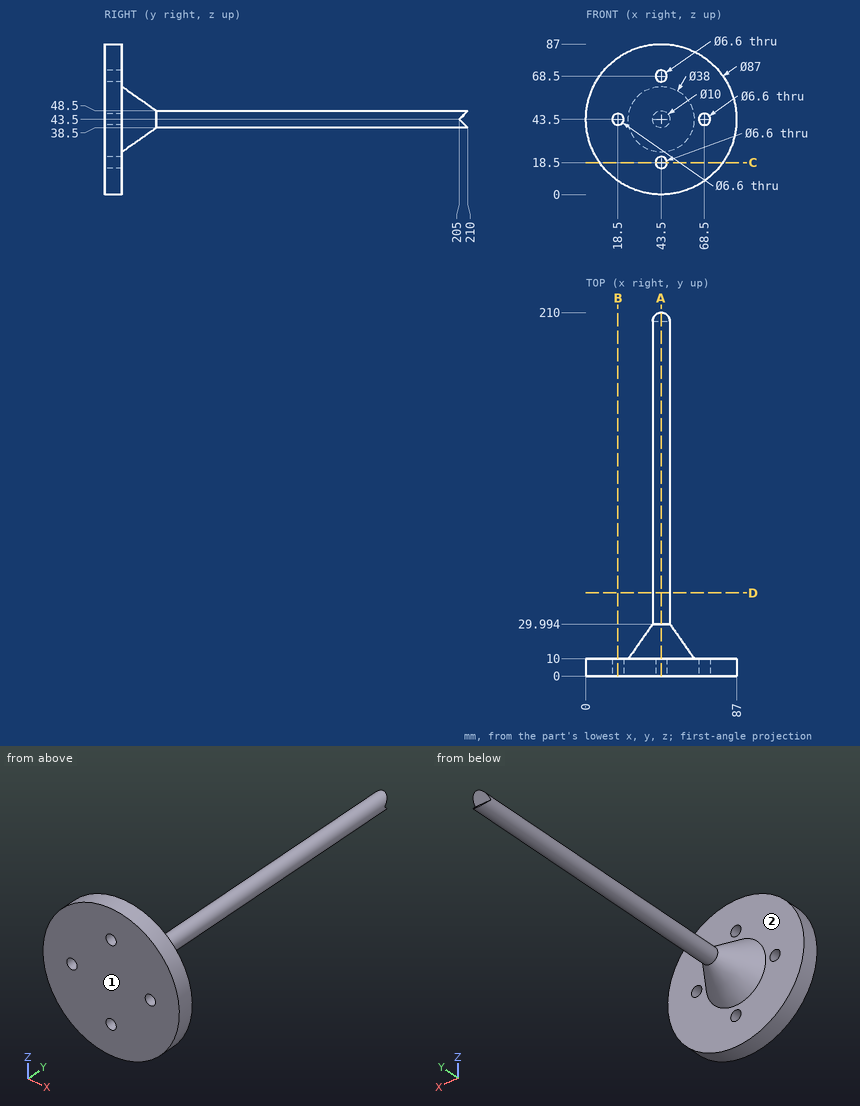
Answer from the drawing. Dimensions are ordinates in mm from the lowest x, y and z of the part. A direction names the side the tool comes from. Coordinates: 2 decimals unless noted, no trailing zeros. Order: outer loops, then holes, each group sorted by start corner. A loop starts at its lowest first (then second) coordinate and runs counter-clockwise, first axis right, second up. Notation, with made-up numbers: M 4,-23.75 L 51,-23.75 A28 cw 51,10.25 Z; hole C 61,-36.5 d1. An arc over 180 degrees is marked long. Put each result on its own line as item: value. Start each with the question number.
Item 1: For the marked faces 1 and 2, determine the directions among +Z, -Z, +X, -X, +Y, -Y from which every point of the face is accessible in a straight line to the end or side of a thin tool.
Item 2: Given pin 1 Ø1 at (x, z) = (73.5, 58) entering from +Y; pin 2 Ø10.5 at (x, z) = (68.5, 43.5) entering from -Y; pin 3 Ø5 at (y, z) = (48, 37.5) entering from -X; pin 4 Ø4 at (x, y) = (42.5, 57.5) entering from +Z, each flat-ended and moving along its own axis, determine where each tip first touches the part or whether it passes through.
Item 3: Section C-C, the plane z = 18.5 is taken. Determine the outline of the cut face in (x, y), plus the area to 3 significant figures.
Item 4: Section D-D, the plane y = 48 is taken. Determine the outline of the cut face in (x, z), plus the area to 3 significant figures.
Item 5: Section B-B, the plane x = 18.5 is taken. Determine the outline of the cut face in (y, z), plus the area to 3 significant figures.
Item 6: Consider probe 1 along Z at (x, y) = (43, 5); probe 2 along Y at (x, z) = (22, 28.5). Determine where each line is inside the solid, lowest interval first. Write a range as [from, to].
Item 7: Section A-A, the plane x = 43.5 is taken. Determine the outline of the cut face in (y, z).
Computed:
1. face 1: +Z, -Z, +X, -X, -Y
1. face 2: +Y
2. pin 1: stops at y = 10
2. pin 2: stops at y = 0
2. pin 3: stops at x = 39.93
2. pin 4: stops at z = 48.5
3. outline: M 7.9,0 L 40.2,0 L 40.2,10 L 7.9,10 Z; M 46.8,0 L 79.1,0 L 79.1,10 L 46.8,10 Z
3. area: 646 mm2
4. outline: C 43.5,43.5 d10
4. area: 78.5 mm2
5. outline: M 0,7.9 L 10,7.9 L 10,40.2 L 0,40.2 Z; M 0,46.8 L 10,46.8 L 10,79.1 L 0,79.1 Z
5. area: 646 mm2
6. probe 1: z = [0, 15.24], [21.76, 65.24], [71.76, 87]
6. probe 2: y = [0, 10]
7. outline: M 0,0 L 10,0 L 10,15.2 L 0,15.2 Z; M 0,21.8 L 10,21.8 L 10,24.5 L 29.99,38.5 L 210,38.5 L 205,43.5 L 210,48.5 L 29.99,48.5 L 10,62.5 L 10,65.2 L 0,65.2 Z; M 0,71.8 L 10,71.8 L 10,87 L 0,87 Z
